Part model, mm, in its own coordinate system. Round coordinates to 2 decimals unless told otherwise and drop trailing zeros. Loops run counter-clockwise (first coordinate to the right, second up) from the corner with the lowest first, then second, coordinate; pieces in that order, holes last.
(1) Cut at B-B on x = 137.5. List the corners of the cut face in (y, z).
(2) Probe probe 1 along X at (y, z) = (-51.5, 168.85); probe 2 along X at (y, z) = (-52.5, 167.8); probe 3 along X at (y, z) = (-92, 168.85). List the from-to ranges inside material, lowest first.
(3) Cut at A-A on z = 168.75. Count the separate pieces of the cut face and the enclosed holes in it, then the cut area to 3 significant figures.
(4) Flat gauge pins, fed straight in: pin 1 (0.8 mm diameter, centred on x = 462.5, z = 168, fed in from -Y); pin 2 (1.3 mm diameter, centred on x = 51.5, z = 168, fed in from +Y); pin 3 (1.5 mm diameter, centred on y = -60.5, z = 169, fed in from +X). Where does each tip first touch, or does it go through?
from build123d import *

# Parameters (mm, degrees)
SKETCH2_R           = 4
SKETCH2_R_2         = 1.651
BOSS_EXTRUDE1_DEPTH = 2.54
FILLET2_R           = 6.35


with BuildPart() as part:
    # Sketch2 → Boss-Extrude1 (new body)
    with BuildSketch(Plane(origin=(33.288009597, -76.684680992, 167.069664602), x_dir=(1, 0, 0), z_dir=(0, 0, 1))):
        with BuildLine():
            ThreePointArc((456.517892766, 21.339609639), (445.792378932, 30.866970077), (435.85, 20.525))
            Line((435.85, 20.525), (421.85, 20.525))
            ThreePointArc((421.85, 20.525), (411.5, 30.875), (401.15, 20.525))
            Line((401.15, 20.525), (62.352851741, 20.525))
            ThreePointArc((62.352851741, 20.525), (52.002851741, 30.875), (41.652851741, 20.525))
            Line((41.652851741, 20.525), (0, 20.525))
            Line((0, 20.525), (0, -7.825))
            Line((0, -7.825), (41.652851741, -7.825))
            ThreePointArc((41.652851741, -7.825), (52.002851741, -18.175), (62.352851741, -7.825))
            Line((62.352851741, -7.825), (401.15, -7.825))
            ThreePointArc((401.15, -7.825), (411.5, -18.175), (421.85, -7.825))
            Line((421.85, -7.825), (435.85, -7.825))
            ThreePointArc((435.85, -7.825), (445.792378932, -18.166970077), (456.517892766, -8.639609639))
            Line((456.517892766, -8.639609639), (457.2, 0))
            Line((457.2, 0), (457.2, 12.7))
            Line((457.2, 12.7), (456.517892766, 21.339609639))
        make_face()
        with Locations((52.002851741, -7.825)):
            Circle(SKETCH2_R, mode=Mode.SUBTRACT)
        with Locations((411.5, -7.825)):
            Circle(SKETCH2_R, mode=Mode.SUBTRACT)
        with Locations((428.85, -1.905)):
            Circle(SKETCH2_R_2, mode=Mode.SUBTRACT)
        with Locations((52.002851741, 20.525)):
            Circle(SKETCH2_R, mode=Mode.SUBTRACT)
        with Locations((428.85, 14.605)):
            Circle(SKETCH2_R_2, mode=Mode.SUBTRACT)
        with Locations((411.5, 20.525)):
            Circle(SKETCH2_R, mode=Mode.SUBTRACT)
        with Locations((446.2, 20.525)):
            Circle(SKETCH2_R, mode=Mode.SUBTRACT)
        with Locations((446.2, -7.825)):
            Circle(SKETCH2_R, mode=Mode.SUBTRACT)
    extrude(amount=BOSS_EXTRUDE1_DEPTH)

    # Fillet2
    fillet2_edges = [part.edges().sort_by_distance(p)[0] for p in [
        (95.640861339, -84.509680992, 168.339664602),
        (74.940861339, -84.509680992, 168.339664602),
        (74.940861339, -56.159680992, 168.339664602),
        (95.640861339, -56.159680992, 168.339664602),
        (434.438009597, -56.159680992, 168.339664602),
        (455.138009597, -56.159680992, 168.339664602),
        (469.138009597, -56.159680992, 168.339664602),
        (469.138009597, -84.509680992, 168.339664602),
        (455.138009597, -84.509680992, 168.339664602),
        (434.438009597, -84.509680992, 168.339664602),
    ]]
    fillet(fillet2_edges, radius=FILLET2_R)


solid = part.part
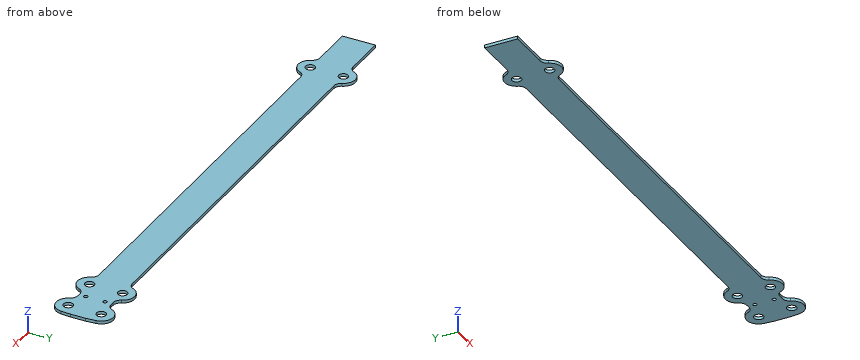
Final values:
1. outline: (-84.51, 167.07) - (-56.16, 167.07) - (-56.16, 169.61) - (-84.51, 169.61) - close
2. probe 1: x = 76.05 to 94.53, 435.55 to 454.03, 470.25 to 488.73
2. probe 2: x = 75.6 to 83.68, 86.91 to 94.98, 435.09 to 443.17, 446.4 to 454.48, 469.79 to 477.87, 481.1 to 489.17
2. probe 3: x = 78.15 to 92.43, 437.65 to 451.93, 472.35 to 486.63
3. separate pieces: 1
3. enclosed holes: 8
3. area: 13,700 mm2
4. pin 1: stops at y = -84.51
4. pin 2: stops at y = -56.16
4. pin 3: stops at x = 490.27
